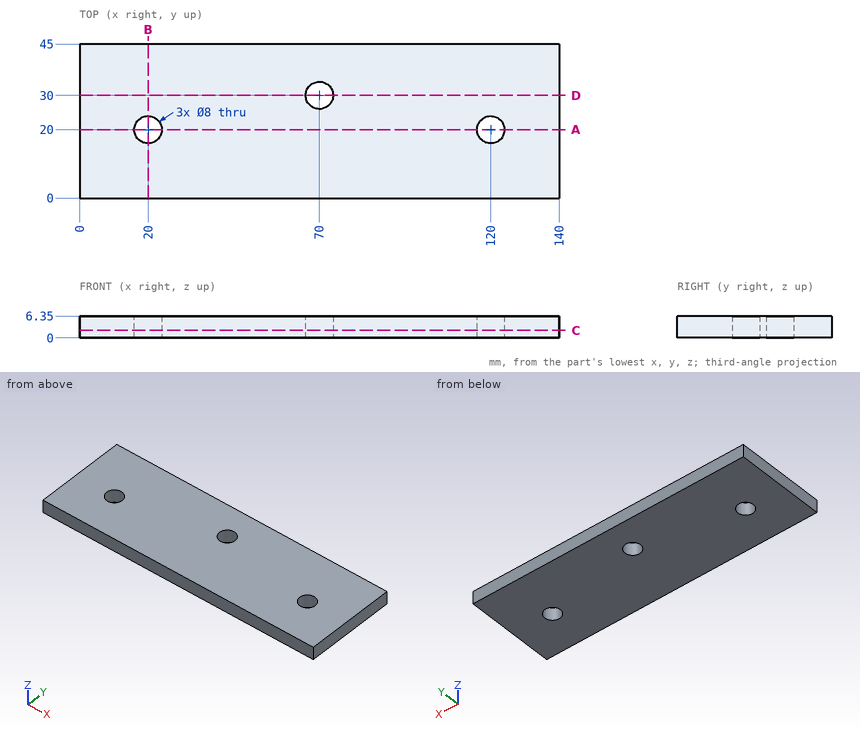
Input: dimensioned drawing with shaded views. Units: mm. Origin: part minimum x, y, z. Round coordinates to 2 decimals unless told otherwise and drop trailing zeros. Order: outer loops, then holes, each group sorted by start corner. A loop starts at its lowest first (then second) coordinate and runs counter-clockwise, first axis right, second up. Notation, with made-up numbers: (16, 43.5) - (27, 43.5) arc R26 cw to (27, 67.5) - close; hole circle Ø1 at (54.25, 71.5). An arc over 180 degrees is marked (long way). Answer as a JSON object with one key per item and string values. Group by question number.
(1) Cut plane A-A (y = 20). Return loops of the section in (x, z), then the cut area to 3 significant figures.
(2) Cut plane D-D (y = 30). Return loops of the section in (x, z).
(3) Material intervals for probe 1 along Y at (x, z) = (20, 2.75); probe 2 along X at (y, z) = (17.5, 0.5); probe 3 along Y at (x, z) = (70, 2.75), sorted ascending. Write a range as from..to.
(4) Cut plane C-C (z = 2.25). Return loops of the section in (x, y).
(5) Cut plane B-B (x = 20). Return loops of the section in (y, z), then the cut area to 3 significant figures.
Here are the results:
{
 "1": {"outline": "(0, 0) - (16, 0) - (16, 6.35) - (0, 6.35) - close; (24, 0) - (116, 0) - (116, 6.35) - (24, 6.35) - close; (124, 0) - (140, 0) - (140, 6.35) - (124, 6.35) - close", "area": "787 mm^2"},
 "2": {"outline": "(0, 0) - (66, 0) - (66, 6.35) - (0, 6.35) - close; (74, 0) - (140, 0) - (140, 6.35) - (74, 6.35) - close"},
 "3": {"probe 1": "y = 0..16, 24..45", "probe 2": "x = 0..16.88, 23.12..116.88, 123.12..140", "probe 3": "y = 0..26, 34..45"},
 "4": {"outline": "(0, 0) - (140, 0) - (140, 45) - (0, 45) - close; hole circle Ø8 at (20, 20); hole circle Ø8 at (70, 30); hole circle Ø8 at (120, 20)"},
 "5": {"outline": "(0, 0) - (16, 0) - (16, 6.35) - (0, 6.35) - close; (24, 0) - (45, 0) - (45, 6.35) - (24, 6.35) - close", "area": "235 mm^2"}
}
